Here's how the part is built. I have some questions about the finished solid (model axes, mm). A direction names the side the tool comes from. Give positions to 0.01 mm unless a question says otherwise; leave off trailing zeros. Loops run counter-clockwise (first coordinate to the right, second up) from the corner with the lowest first, then second, coordinate; pieces in that order, holes last. Notation, with made-up numbers: M -3,29 L 16,29 A17 ccw 16,42 Z; hole C 24,-13 d11. An arc over 180 degrees is marked long. Write item = value, one per line. Start each with the question number.
```python
from build123d import *

# Parameters (mm, degrees)
F1_DEPTH = 63.5
F2_W     = 38.1
F2_H     = 25.4
F3_DEPTH = 50.8


with BuildPart() as f1:
    # F0 (on Front) → F1 (new body)
    with BuildSketch(Plane.XZ):
        Polygon((2.150557, 8.363415), (-61.349443, 8.363415), (-61.349443, -17.036585), (-23.249443, -17.036585), (-23.249443, -67.836585), (52.950557, -67.836585), (52.950557, -42.436585), (2.150557, -42.436585), align=None)
    extrude(amount=-F1_DEPTH)

    # F2 (on face) → F3 (join)
    with BuildSketch(Plane.XY.offset(-42.436585)):
        with Locations((21.200557, 50.8)):
            Rectangle(F2_W, F2_H)
    extrude(amount=F3_DEPTH)


solid = f1.part
```
Q1. If we section it at B-B, the plane x = 17: List the corners of the cut face in (y, z) for me.
Q2. If we section it at A-A, the plane y = 42: List the corners of the cut face in (x, z) for me.
Q3. If we section it at D-D, the plane y = 35.5: List the corners of the cut face in (x, z) for me, then the cut area to 3 significant figures.
Q4. If I drill on line 1 along Z through (x, y) = (-45, 24.5); line 2 along X through (y, z) = (54.5, -7); line 3 along Z through (x, y) = (30.5, 14), over which ranges is the centre line in solid material (lowest first)?
Q5. Will these pins go through, and if not, where does the flat tip stop? pin 1 (11.5 mm diameter, centred on y = 13.5, z = -21.5, fed in from +X); pin 2 (6 mm diameter, centred on y = 54.5, z = -23, fed in from +X); pin 3 (8 mm diameter, centred on y = 26.5, z = -53.5, fed in from -X).
Q6. On a 3-axis mill with a long thin cutter (end or side, diameter ignored), from which of +Z, -Z, +X, -X, +Y, -Y can I reach the whole of each face in a straight line? I mean faces 1 (the flat face through (-43, 31, -17.037)), 2 (the flat face through (-5, 0, -29)), 3 (the flat face through (8, 63.5, -30)), 4 (the flat face through (40.251, 51, -17)), 5 (the flat face through (21, 38.1, -17)). Say none if no direction works.
Q7. If we section it at C-C, the plane z = -26.5: List the corners of the cut face in (x, y) for me, then the cut area to 3 significant figures.
Resolved:
q1.outline = M 0,-67.84 L 63.5,-67.84 L 63.5,8.36 L 38.1,8.36 L 38.1,-42.44 L 0,-42.44 Z
q2.outline = M -61.35,-17.04 L -23.25,-17.04 L -23.25,-67.84 L 52.95,-67.84 L 52.95,-42.44 L 40.25,-42.44 L 40.25,8.36 L -61.35,8.36 Z
q3.outline = M -61.35,-17.04 L -23.25,-17.04 L -23.25,-67.84 L 52.95,-67.84 L 52.95,-42.44 L 2.15,-42.44 L 2.15,8.36 L -61.35,8.36 Z
q3.area = 4,190 mm²
q4.line_1 = -17.04 to 8.36
q4.line_2 = -61.35 to 40.25
q4.line_3 = -67.84 to -42.44
q5.pin_1 = 2.15
q5.pin_2 = 40.25
q5.pin_3 = -23.25
q6.face_1 = -Z, -X, +Y, -Y
q6.face_2 = +Z, -Z, +X, -X, -Y
q6.face_3 = +Z, -Z, +X, -X, +Y
q6.face_4 = +Z, +X, +Y, -Y
q6.face_5 = +Z, +X, -Y
q7.outline = M -23.25,0 L 2.15,0 L 2.15,38.1 L 40.25,38.1 L 40.25,63.5 L -23.25,63.5 Z
q7.area = 2,580 mm²
